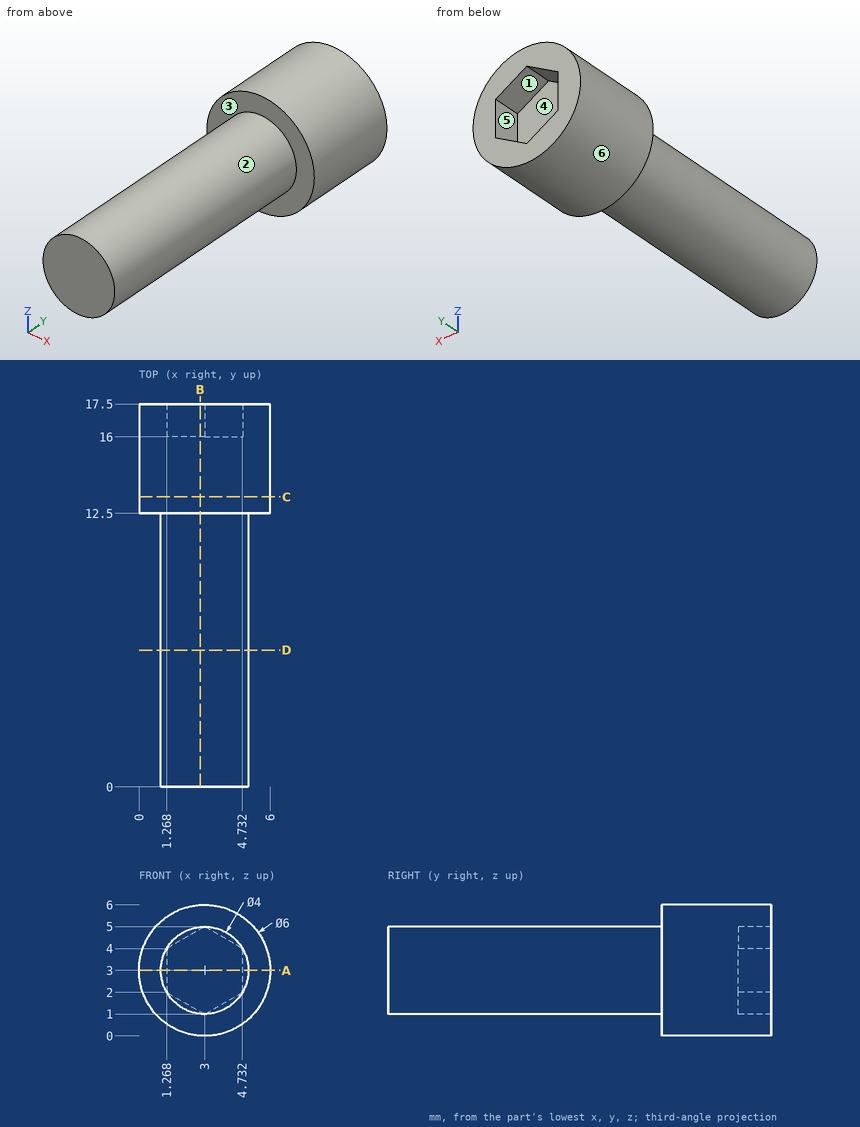
Job drawing, mm, ordinate dimensions from the low corner. One solid piece. A direction names the side the tool comes from. Round coordinates to 2 decimals unless told otherwise and drop trailing zeros. Loops run counter-clockwise (first coordinate to the right, second up) from the corner with the lowest first, then second, coordinate; pieces in that order, holes last.
Item 1: Mould opens along Z. For the marked faces 1, 2, 3 and 4 say: +Z half, -Z half, draft (parallel to the pull), parting line (faces both ways), or undercut.
Item 2: Drill centre lines: line 1 (Y direction, x = 3.1, z = 3.15); line 2 (Y direction, x = 4.35, z = 4.7); line 3 (X direction, y = 10.25, z = 2.9). Where is each one in solid material? Low to high.
Item 3: Cut at C-C, the plane y = 13.25. Give the cut face in (x, z), then the cut area to 3 significant figures.
Item 4: Drop flat-ended pins along their axis: P1, Ø1, axis at x = 3, z = 2.5, coming from the +Y side; P2, Ø1, axis at y = 6.5, z = 4.5, coming from the +X side; P3, Ø3, axis at x = 4, y = 9.5, coming from the -Z side. Give the stop position or say it passes through.
Item 5: Cut at A-A, the plane z = 3. Give the cut face in (x, y), then the cut area to 3 significant figures.
Item 6: Cut at D-D, the plane y = 6.25. Give the cut face in (x, z).
Item 7: 3-axis set-ups, long thin cutter, end or side, ignore diameter. For the marked faces 5 and 6: which of +Z, -Z, +X, -X, +Y, -Y reach the whole face in a straight line?
Item 8: Cut at B-B, the plane x = 2.8. Give the cut face in (y, z).
A:
1. face 1: undercut
1. face 2: parting line
1. face 3: draft
1. face 4: undercut
2. line 1: y = 0 to 16
2. line 2: y = 12.5 to 17.5
2. line 3: x = 1 to 5
3. outline: circle Ø6 at (3, 3)
3. area: 28.3 mm2
4. P1: stops at y = 16
4. P2: stops at x = 4.73
4. P3: stops at z = 1
5. outline: (0, 12.5) - (1, 12.5) - (1, 0) - (5, 0) - (5, 12.5) - (6, 12.5) - (6, 17.5) - (4.73, 17.5) - (4.73, 16) - (1.27, 16) - (1.27, 17.5) - (0, 17.5) - close
5. area: 74.8 mm2
6. outline: circle Ø4 at (3, 3)
7. face 5: +Y
7. face 6: +Y, -Y
8. outline: (0, 1.01) - (12.5, 1.01) - (12.5, 0.01) - (17.5, 0.01) - (17.5, 1.12) - (16, 1.12) - (16, 4.88) - (17.5, 4.88) - (17.5, 5.99) - (12.5, 5.99) - (12.5, 4.99) - (0, 4.99) - close
